from build123d import *

# Parameters (mm, degrees)
CROQUIS1_W              = 600
CROQUIS1_H              = 200
SALIENTE_EXTRUIR1_DEPTH = 3
CROQUIS2_W              = 3
CROQUIS2_H              = 29.2
CROQUIS2_W_2            = 24.85
CROQUIS2_H_2            = 3
CROQUIS2_W_3            = 49.7
CORTAR_EXTRUIR1_DEPTH   = 4
CORTAR_EXTRUIR2_DEPTH   = 4


with BuildPart() as part:
    # Croquis1 → Saliente-Extruir1 (new body)
    with BuildSketch(Plane.XY):
        Rectangle(CROQUIS1_W, CROQUIS1_H)
    extrude(amount=SALIENTE_EXTRUIR1_DEPTH)

    # Croquis2 → Cortar-Extruir1 (cut, through all)
    with BuildSketch(Plane(origin=(0, 0, 0), x_dir=(-1, 0, 0), z_dir=(0, 0, -1))):
        with Locations((-298.5, 69)):
            Rectangle(CROQUIS2_W, CROQUIS2_H)
        with Locations((298.5, 69)):
            Rectangle(CROQUIS2_W, CROQUIS2_H)
        with Locations((-298.5, 24)):
            Rectangle(CROQUIS2_W, CROQUIS2_H)
        with Locations((298.5, 24)):
            Rectangle(CROQUIS2_W, CROQUIS2_H)
        with Locations((-298.5, -21)):
            Rectangle(CROQUIS2_W, CROQUIS2_H)
        with Locations((298.5, -21)):
            Rectangle(CROQUIS2_W, CROQUIS2_H)
        with Locations((-298.5, -66)):
            Rectangle(CROQUIS2_W, CROQUIS2_H)
        with Locations((298.5, -66)):
            Rectangle(CROQUIS2_W, CROQUIS2_H)
        with Locations((-287.575, -98.5)):
            Rectangle(CROQUIS2_W_2, CROQUIS2_H_2)
        with Locations((287.575, -98.5)):
            Rectangle(CROQUIS2_W_2, CROQUIS2_H_2)
        with Locations((-200, -98.5)):
            Rectangle(CROQUIS2_W_3, CROQUIS2_H_2)
        with Locations((200, -98.5)):
            Rectangle(CROQUIS2_W_3, CROQUIS2_H_2)
        with Locations((-100, -98.5)):
            Rectangle(CROQUIS2_W_3, CROQUIS2_H_2)
        with Locations((100, -98.5)):
            Rectangle(CROQUIS2_W_3, CROQUIS2_H_2)
        with Locations((0, -98.5)):
            Rectangle(CROQUIS2_W_3, CROQUIS2_H_2)
    extrude(amount=-CORTAR_EXTRUIR1_DEPTH, mode=Mode.SUBTRACT)

    # Croquis3 → Cortar-Extruir2 (cut, through all)
    with BuildSketch(Plane.XY.offset(3)):
        with BuildLine():
            ThreePointArc((-163.5, 77), (-160, 73.5), (-156.5, 77))
            ThreePointArc((-156.5, 77), (-160, 80.5), (-163.5, 77))
        make_face()
        with BuildLine():
            ThreePointArc((-133.45, 83.4), (-129.95, 79.9), (-126.45, 83.4))
            ThreePointArc((-126.45, 83.4), (-129.95, 86.9), (-133.45, 83.4))
        make_face()
        with BuildLine():
            ThreePointArc((126.45, 83.4), (129.95, 79.9), (133.45, 83.4))
            ThreePointArc((133.45, 83.4), (129.95, 86.9), (126.45, 83.4))
        make_face()
        with BuildLine():
            ThreePointArc((156.5, 77), (160, 73.5), (163.5, 77))
            ThreePointArc((163.5, 77), (160, 80.5), (156.5, 77))
        make_face()
        with BuildLine():
            ThreePointArc((186.55, 83.4), (190.05, 79.9), (193.55, 83.4))
            ThreePointArc((193.55, 83.4), (190.05, 86.9), (186.55, 83.4))
        make_face()
        with BuildLine():
            ThreePointArc((-193.55, 83.4), (-190.05, 79.9), (-186.55, 83.4))
            ThreePointArc((-186.55, 83.4), (-190.05, 86.9), (-193.55, 83.4))
        make_face()
    extrude(amount=-CORTAR_EXTRUIR2_DEPTH, mode=Mode.SUBTRACT)


solid = part.part
Check sheet for the modelled part. Datum: model origin and axes. Units: mm. Round coordinates to 2 decimals unless told otherwise and drop trailing zeros. Answer as CSV lines item,"result". Start each with the question number.
1) Material ranges on line 1 (Y direction, x = 160, z = 0.95); line 2 (Y direction, x = 190.05, z = 1.4); line 3 (X direction, y = 29.5, z = 2.3), recorded low to high. Write a range as from..to.
2) Section check A-A on z = 0.75. State how many separate pieces and enclosed holes the cut face has, and give its area (3 significant figures).
3) Go/stop test with flat-tipped pins: P1, Ø0.9, axis at x = 299, z = 1, coming from the -Y side; P2, Ø0.9, axis at y = -99, z = 2, coming from the -X side; P3, Ø4, axis at x = 129.95, y = 83.4, coming from the +Z side; P4, Ø1.5, axis at y = -27.5, z = 2, coming from the +X side. Record where each tip stops, or that it passes through.
Found:
1,line 1,"y = -100..73.5, 80.5..100"
1,line 2,"y = -97..79.9, 86.9..100"
1,line 3,"x = -297..297"
2,separate pieces,"1"
2,enclosed holes,"6"
2,area,"118,000 mm^2"
3,P1,"stops at y = -97"
3,P2,"stops at x = -275.15"
3,P3,"passes through"
3,P4,"stops at x = 297"
